Work out the finished part from the listing and answer in its coordinate system (mm). Face numbers are marked on the shaded views. A direction names the side the tool comes from. Round coordinates to 2 decimals unless told otherwise and drop trailing zeros. Write each loop counter-clockwise with the first axis right and the second up, starting at its lowest first coordinate (ties: lowest second). Pieces come first, ordered by that corner, then holes. Notation, with made-up numbers: (58.25, -29) - (106.25, -29) arc R15 ccw to (106.25, -15) - close; hole circle Ø5 at (45.5, -10.5). An arc over 180 degrees is marked (long way). Answer as a JSON object with one key per item and string values.
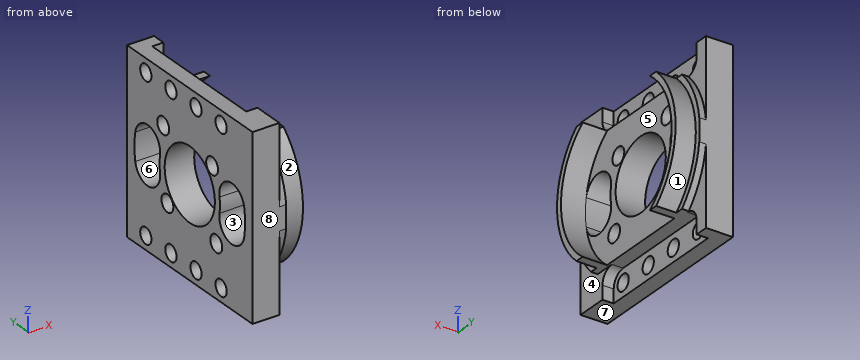
Autodesk Inventor part; units mm, degrees
ref_plane "YZ Plane" through (0, 0, 0) normal (1, 0, 0) x (0, 1, 0)
ref_plane "XZ Plane" through (0, 0, 0) normal (0, 1, 0) x (-1, 0, 0)
ref_plane "XY Plane" through (0, 0, 0) normal (0, 0, 1) x (1, 0, 0)
sketch "Sketch4" plane through (0, 0, 0) normal (1, 0, 0) x (0, 1, 0)
  line L0 (15.875, 15.875) -> (-15.875, 15.875)
  line L1 (-15.875, 15.875) -> (-15.875, -15.875)
  line L2 (-15.875, -15.875) -> (15.875, -15.875)
  line L3 (15.875, -15.875) -> (15.875, 15.875)
  line L4 (15.875, 15.875) -> (-15.875, -15.875) construction
  line L5 (-15.875, 15.875) -> (15.875, -15.875) construction
  circle A0 centre (0, 0) radius 6.35
  line L6 (0, 0) -> (0, 15.875) construction
  line L7 (0, 22.4506) -> (-22.4506, 0)
  line L8 (-22.4506, 0) -> (0, -22.4506)
  line L9 (0, -22.4506) -> (22.4506, 0)
  line L10 (22.4506, 0) -> (0, 22.4506)
  line L11 (0, 22.4506) -> (0, -22.4506) construction
  line L12 (-22.4506, 0) -> (22.4506, 0) construction
  point P0 (15.875, 6.5756)
  point P1 (6.5756, 15.875)
  point P2 (-6.5756, 15.875)
  point P3 (-15.875, 6.5756)
  point P4 (-15.875, -6.5756)
  point P5 (-6.5756, -15.875)
  point P6 (6.5756, -15.875)
  point P7 (15.875, -6.5756)
  dimension "d37" = 31.75
  dimension "d38" = 31.75
  dimension "d39" = 12.7
  dimension "d126" = 31.75
  dimension "d127" = 31.75
  dimension "d128" = 45
extrude "Extrusion5" add sketch "Sketch4" along normal blind 9.525 contours L3 L10 L0 | L10 L3 L9 L2 L8 L1 L7 L0 | L7 L1 L0 | L3 L2 L9 | L8 L2 L1
sketch "Sketch5" plane through (9.525, 0, 0) normal (1, 0, 0) x (0, 0, -1)
  circle A0 centre (0, 0) radius 25.4
  circle A1 centre (0, 0) radius 15
  circle A2 centre (0, 0) radius 14
  circle A3 centre (0, 0) radius 16
  dimension "d50" = 50.8
  dimension "d51" = 30
  dimension "d52" = 1
  dimension "d55" = 1
extrude "Extrusion6" cut sketch "Sketch5" against normal blind 3.5719 contours A0 | A3
extrude "Extrusion7" cut sketch "Sketch5" against normal blind 4.7625 contours A0
sketch "Sketch7" plane through (9.525, 0, 0) normal (1, 0, 0) x (0, 0, -1)
  circle A0 centre (0, 0) radius 14
  circle A1 centre (0, 0) radius 15
  dimension "d97" = 1
extrude "Extrusion10" cut sketch "Sketch7" against normal blind 4.3094 contours A0
sketch "Sketch8" plane through (5.2156, 0, 0) normal (1, 0, 0) x (0, 0, -1)
  circle A0 centre (0, 0) radius 8 construction
  line L0 (0, 0) -> (8, 0) construction
  line L1 (0, 0) -> (5.6569, 5.6569) construction
  circle A1 centre (5.6569, 5.6569) radius 1.5
  circle A2 centre (0, 0) radius 9.5 construction
  line L2 (0, 0) -> (6.7175, -6.7175) construction
  circle A3 centre (6.7175, -6.7175) radius 1.5
  circle A4 centre (-6.7175, 6.7175) radius 1.5
  circle A5 centre (-5.6569, -5.6569) radius 1.5
  arc A6 (-1.8797, -10.6605) -> (1.8797, -10.6605) centre (0, 0) ccw construction
  arc A7 (-2.4311, -13.7873) -> (2.4311, -13.7873) centre (0, 0) ccw
  arc A8 (-1.3284, -7.5338) -> (1.3284, -7.5338) centre (0, 0) ccw
  arc A9 (-1.3284, -7.5338) -> (-2.4311, -13.7873) centre (-1.8797, -10.6605) ccw
  arc A10 (2.4311, -13.7873) -> (1.3284, -7.5338) centre (1.8797, -10.6605) ccw
  circle A11 centre (0, 0) radius 14
  line L3 (0, -10.825) -> (0, 0) construction
  line L4 (1.8797, -10.6605) -> (0, 0) construction
  arc A12 (1.8797, 10.6605) -> (-1.8797, 10.6605) centre (0, 0) ccw construction
  arc A13 (-2.4311, 13.7873) -> (-1.3284, 7.5338) centre (-1.8797, 10.6605) ccw
  arc A14 (2.4311, 13.7873) -> (-2.4311, 13.7873) centre (0, 0) ccw
  arc A15 (1.3284, 7.5338) -> (2.4311, 13.7873) centre (1.8797, 10.6605) ccw
  arc A16 (1.3284, 7.5338) -> (-1.3284, 7.5338) centre (0, 0) ccw
  point P0 (0, 10.825)
  point P1 (2.4311, 13.7873)
  point P2 (-2.4311, 13.7873)
  dimension "d150" = 19
  dimension "d70" = 16
  dimension "d71" = 3
  dimension "d72" = 45
  dimension "d151" = 3
  dimension "d154" = 360
  dimension "d169" = 3.175
  dimension "d170" = 45
  dimension "d171" = 10
  dimension "d174" = 360
extrude "Extrusion11" cut sketch "Sketch8" along normal through all both and the other way through all contours A1 | A3 | A4 | A5 | A9 A8 A10 A7 | A11 A15 A16 A13
sketch "Sketch14" plane through (9.525, 0, 0) normal (1, 0, 0) x (0, 0, -1)
  line L0 (15.875, -15.875) -> (15.875, 15.875)
  line L1 (-15.875, -15.875) -> (15.875, -15.875)
  line L2 (15.875, 15.875) -> (11.1125, 15.875)
  line L3 (11.1125, 15.875) -> (11.1125, -15.875)
  line L4 (11.1125, -15.875) -> (15.875, -15.875)
  line L5 (15.875, -15.875) -> (15.875, 15.875)
  line L6 (15.875, 15.875) -> (-15.875, 15.875)
  line L7 (-1.9961, -15.875) -> (-15.875, -15.875)
  line L8 (-15.875, 15.875) -> (-11.1125, 15.875)
  line L9 (-11.1125, 15.875) -> (-11.1125, -15.875)
  line L10 (-11.1125, -15.875) -> (-15.875, -15.875)
  line L11 (-15.875, -15.875) -> (-15.875, 15.875)
  point P0 (0, 0)
  point P1 (-11.1125, -15.875)
  dimension "d206" = 4.7625
  dimension "d207" = 4.7625
extrude "Extrusion17" cut sketch "Sketch14" against normal up to surface (4.7625 mm away) contours L1 L3 L2 L0 | L9 L1 L11 L6
sketch "Sketch15" plane through (9.525, 0, 0) normal (1, 0, 0) x (0, 0, -1)
  line L0 (15.875, -15.875) -> (15.875, 15.875)
  line L1 (15.875, 13.4938) -> (11.1125, 13.4938)
  line L2 (11.1125, 13.4938) -> (11.1125, -13.4938)
  line L3 (11.1125, -13.4938) -> (15.875, -13.4938)
  line L4 (15.875, -13.4938) -> (15.875, 13.4938)
  line L5 (-1.9961, 15.875) -> (1.9961, 15.875)
  line L6 (0, 15.875) -> (0, -15.875) construction
  line L7 (-15.875, -15.875) -> (15.875, -15.875)
  line L8 (13.4938, 13.4938) -> (13.4938, -13.4938) construction
  circle A0 centre (13.4938, 11.1125) radius 1.4224
  circle A1 centre (13.4938, 4.7625) radius 1.4224
  circle A2 centre (13.4938, -1.5875) radius 1.4224
  circle A3 centre (13.4938, -7.9375) radius 1.4224
  line L9 (15.875, 0) -> (11.1125, 0) construction
  line L10 (-15.875, 13.4938) -> (-11.1125, 13.4938)
  line L11 (-11.1125, 13.4938) -> (-11.1125, -13.4938)
  line L12 (-11.1125, -13.4938) -> (-15.875, -13.4938)
  line L13 (-15.875, -13.4938) -> (-15.875, 13.4938)
  line L14 (-13.4938, 13.4938) -> (-13.4938, -13.4938) construction
  circle A4 centre (-13.4938, 11.1125) radius 1.4224
  circle A5 centre (-13.4938, 4.7625) radius 1.4224
  circle A6 centre (-13.4938, -1.5875) radius 1.4224
  circle A7 centre (-13.4938, -7.9375) radius 1.4224
  line L15 (-15.875, 0) -> (-11.1125, 0) construction
  point P0 (0, 0)
  point P1 (0, 0)
  dimension "d210" = 4.7625
  dimension "d211" = 26.9875
  dimension "d212" = 2.8448
  dimension "d213" = 2.3813
  dimension "d216" = 6.35
extrude "Extrusion18" cut sketch "Sketch15" against normal through all contours A0 | A1 | A2 | A3 | A4 | A5 | A6 | A7
sketch "Sketch16" plane through (5.9531, 0, 0) normal (1, 0, 0) x (0, 0, -1)
  circle A0 centre (-13.4938, -1.5875) radius 1.4224 construction
  circle A1 centre (-13.4938, 4.7625) radius 1.4224 construction
  circle A2 centre (-13.4938, -7.9375) radius 1.4224 construction
  circle A3 centre (-13.4938, 11.1125) radius 1.4224 construction
  line L0 (-1.9961, -15.875) -> (-15.875, -15.875) construction
  arc A4 (-11.1125, -11.5114) -> (-1.9961, -15.875) centre (0, 0) ccw construction
  line L1 (-11.1125, 11.5114) -> (-11.1125, -11.5114)
  arc A5 (-1.9961, 15.875) -> (-11.1125, 11.5114) centre (0, 0) ccw construction
  line L2 (-15.875, 15.875) -> (-1.9961, 15.875) construction
  line L3 (-15.875, -15.875) -> (-15.875, 15.875) construction
  circle A6 centre (13.4938, 4.7625) radius 1.4224 construction
  circle A7 centre (13.4938, -1.5875) radius 1.4224 construction
  circle A8 centre (13.4938, 11.1125) radius 1.4224 construction
  circle A9 centre (13.4938, -7.9375) radius 1.4224 construction
  line L4 (1.9961, 15.875) -> (15.875, 15.875) construction
  arc A10 (11.1125, 11.5114) -> (1.9961, 15.875) centre (0, 0) ccw construction
  line L5 (11.1125, -11.5114) -> (11.1125, 11.5114)
  arc A11 (1.9961, -15.875) -> (11.1125, -11.5114) centre (0, 0) ccw construction
  line L6 (15.875, -15.875) -> (1.9961, -15.875) construction
  line L7 (15.875, 15.875) -> (15.875, -15.875) construction
  circle A12 centre (-13.4938, -7.9375) radius 2.3812
  circle A13 centre (-13.4938, -1.5875) radius 2.3812
  circle A14 centre (-13.4938, 4.7625) radius 2.3812
  circle A15 centre (-13.4938, 11.1125) radius 2.3812
  circle A16 centre (13.4938, -7.9375) radius 2.3812
  circle A17 centre (13.4938, -1.5875) radius 2.3812
  circle A18 centre (13.4938, 4.7625) radius 2.3812
  circle A19 centre (13.4938, 11.1125) radius 2.3812
  line L8 (15.875, 15.875) -> (15.875, -15.875)
  line L9 (13.4938, 13.4937) -> (15.875, 13.4937)
  line L10 (15.875, 13.4937) -> (15.875, -10.3188)
  line L11 (15.875, -10.3188) -> (13.4938, -10.3188)
  line L12 (13.4938, -10.3188) -> (13.4938, 13.4937) construction
  line L13 (-15.875, -15.875) -> (-15.875, 15.875)
  line L14 (-13.4938, 13.4937) -> (-15.875, 13.4937)
  line L15 (-15.875, 13.4937) -> (-15.875, -10.3188)
  line L16 (-15.875, -10.3188) -> (-13.4938, -10.3188)
  line L17 (-13.4938, -10.3188) -> (-13.4938, 13.4937) construction
  point P0 (-15.875, -7.9375)
  point P1 (-15.875, -1.5875)
  point P2 (-11.1125, -7.9375)
  point P3 (-11.1125, -1.5875)
  point P4 (-15.875, 4.7625)
  point P5 (-11.1125, 4.7625)
  point P6 (-15.875, 11.1125)
  point P7 (-11.1125, 11.1125)
  point P8 (15.875, -7.9375)
  point P9 (15.875, -1.5875)
  point P10 (11.1125, -1.5875)
  point P11 (11.1125, -7.9375)
  point P12 (15.875, 4.7625)
  point P13 (11.1125, 4.7625)
  point P14 (15.875, 11.1125)
  point P15 (11.1125, 11.1125)
  dimension "d223" = 4.7625
  dimension "d224" = 6.35
  dimension "d225" = 26.9875
  dimension "d228" = 6.35
  dimension "d231" = 26.9875
extrude "Extrusion19" cut sketch "Sketch16" against normal blind 3.175
equation "\"d37\" = d38"
equation "\"d126\" = d37"
equation "\"d127\" = d126"
properties part number "Motor Plate" material "Aluminum 6061"
Item 1: A cutting plane is placed at B-B (y = 2.5). Write down the section's boundary in (x, z) (1 decimal).
Results found:
{"outline": "(0, -15.9) - (2.8, -15.9) - (2.8, -11.1) - (5.2, -11.1) - (5.2, -5.8) - (0, -5.8) - close; (0, 5.8) - (5.2, 5.8) - (5.2, 11.1) - (2.8, 11.1) - (2.8, 15.9) - (0, 15.9) - close"}
Item 2: A cutting plane is placed at D-D (y = 10.5). Write down the section's boundary in (x, z) (1 decimal), and give its area (3 significant figures).
Results found:
{"outline": "(0, -15.9) - (2.8, -15.9) - (2.8, -14.8) - (0, -14.8) - close; (0, -12.2) - (2.8, -12.2) - (2.8, -11.1) - (6, -11.1) - (6, -10.7) - (9.5, -10.7) - (9.5, -9.3) - (5.2, -9.3) - (5.2, -5.1) - (0, -5.1) - close; (0, 5.1) - (5.2, 5.1) - (5.2, 9.3) - (9.5, 9.3) - (9.5, 10.7) - (6, 10.7) - (6, 11.1) - (2.8, 11.1) - (2.8, 12.2) - (0, 12.2) - close; (0, 14.8) - (2.8, 14.8) - (2.8, 15.9) - (0, 15.9) - close", "area": "88.5 mm²"}
Item 3: A cutting plane is placed at A-A (z = 0). Write down the section's boundary in (x, y) (3 decimals), and give its area (3 significant figures).
Results found:
{"outline": "(0, -15.875) - (5.953, -15.875) - (5.953, -15) - (9.525, -15) - (9.525, -14) - (0, -14) - close; (0, -7.65) - (5.216, -7.65) - (5.216, -6.35) - (0, -6.35) - close; (0, 6.35) - (5.216, 6.35) - (5.216, 7.65) - (0, 7.65) - close; (0, 14) - (9.525, 14) - (9.525, 15) - (5.953, 15) - (5.953, 15.875) - (0, 15.875) - close", "area": "43.0 mm²"}
Item 4: Consider line 1 along Z through (x, y) = (1.75, -5) (3 decimals); line 2 along Y through (x, z) = (4.5, -2) (3 decimals); line 3 along Z through (x, y) = (3, -10.5) (3 decimals). Determine where each line is inside the solid, lowest interval first.
Results found:
{"line 1": "-15.875 to -3.914, 3.914 to 4.308, 7.005 to 15.875", "line 2": "-15.875 to -13.856, -7.488 to -6.027, 6.027 to 7.488, 13.856 to 15.875", "line 3": "-15.875 to -5.051, 5.051 to 15.875"}
Item 5: Determine the mould class of the marked faces 6, 7 and 8 for opening direction Z: pulls with the +Z half, pulls with the -Z half, needs draft (parallel to the pull), parting line crosses it, or undercut.
Results found:
{"face 6": "undercut", "face 7": "pulls with the -Z half", "face 8": "needs draft"}
Item 6: A cutting plane is placed at C-C (z = 14). Write down the section's boundary in (x, y) (1 decimal).
Results found:
{"outline": "(0, -15.9) - (4.8, -15.9) - (4.8, -10.3) - (2.8, -10.3) - (2.8, -9.3) - (0, -9.3) - close; (0, -6.6) - (2.8, -6.6) - (2.8, -2.9) - (0, -2.9) - close; (0, -0.3) - (2.8, -0.3) - (2.8, 3.4) - (0, 3.4) - close; (0, 6.1) - (2.8, 6.1) - (2.8, 9.8) - (0, 9.8) - close; (0, 12.4) - (2.8, 12.4) - (2.8, 13.5) - (4.8, 13.5) - (4.8, 15.9) - (0, 15.9) - close"}
Item 7: For the marked faces 1, 2, 3, 4 and 5, determine the directions among +Z, -Z, +X, -X, +Y, -Y from which every point of the face is accessible in a straight line to the end or side of a thin tool.
Results found:
{"face 1": "+X, +Y", "face 2": "+X, -Y", "face 3": "+X, -X", "face 4": "-Z, +X, -Y", "face 5": "+X"}
Item 8: Each of these flat-tipped pins is pushed along its axis until it touches: P1, Ø4.5, axis at y = 11.11, z = 13.49, coming from the +X side; P2, Ø1, axis at x = 7.5, z = 5.5, coming from the +Y side; P3, Ø11, axis at y = 0.5, z = 3, coming from the +X side. Where does it stop, or does it pass through?
Results found:
{"P1": "x = 2.78", "P2": "y = 14.14", "P3": "x = 5.22"}
